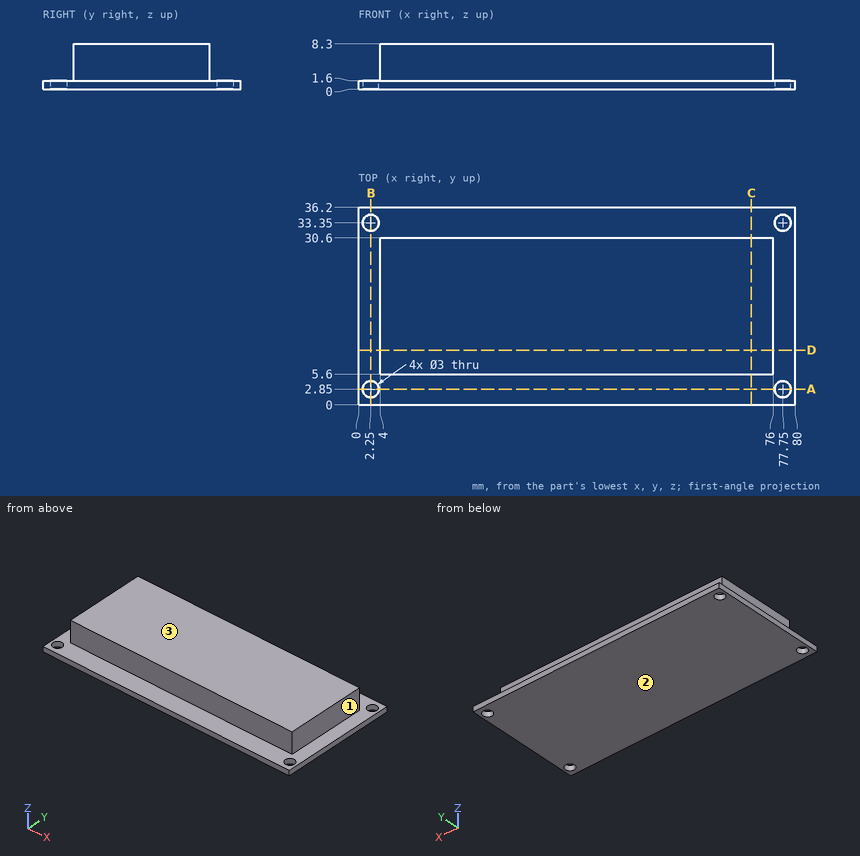
Job drawing, mm, ordinate dimensions from the low corner. One solid piece. Round coordinates to 2 decimals unless told otherwise and drop trailing zeros. Loops run counter-clockwise (first coordinate to the right, second up) from the corner with the lowest first, then second, coordinate; pieces in that order, holes last.
(1) Cut at D-D (y = 10). Give the cut face in (x, z), plus the area to 3 significant figures.
(2) Cut at A-A (y = 2.85). Give the cut face in (x, z).
(3) Drop flat-ended pins along their axis: pin 1 (3.5 mm diameter, centred on x = 2.25, y = 2.85, fed in from +Z); pin 2 (3.5 mm diameter, centred on y = 12.5, z = 3.5, fed in from +X); pin 3 (1 mm diameter, centred on x = 28.5, z = 4.5, fed in from +Y). Give the stop position or say it passes through.
(4) Wall check: line 1 along X through (y, z) = (2.85, 1.3); line 2 along Y through (x, z) = (77.75, 0.65); line 3 along Y through (x, z) = (15, 5.75). Give the ranges that are in metal, low to high.
(5) Cut at B-B (x = 2.25). Give the cut face in (y, z), plus the area to 3 significant figures.
(6) Cut at C-C (x = 72). Give the cut face in (y, z), plus the area to 3 significant figures.
(7) Two-plate mould, pull along Z, no slides. Class the marked faces 1, 2 and 3: +Z half, -Z half, draft (parallel to the pull), parting line (faces both ways), or undercut.
Findings below:
1. outline: (0, 0) - (80, 0) - (80, 1.6) - (76, 1.6) - (76, 8.3) - (4, 8.3) - (4, 1.6) - (0, 1.6) - close
1. area: 610 mm2
2. outline: (0, 0) - (0.75, 0) - (0.75, 1.6) - (0, 1.6) - close; (3.75, 0) - (76.25, 0) - (76.25, 1.6) - (3.75, 1.6) - close; (79.25, 0) - (80, 0) - (80, 1.6) - (79.25, 1.6) - close
3. pin 1: stops at z = 1.6
3. pin 2: stops at x = 76
3. pin 3: stops at y = 30.6
4. line 1: x = 0 to 0.75, 3.75 to 76.25, 79.25 to 80
4. line 2: y = 0 to 1.35, 4.35 to 31.85, 34.85 to 36.2
4. line 3: y = 5.6 to 30.6
5. outline: (0, 0) - (1.35, 0) - (1.35, 1.6) - (0, 1.6) - close; (4.35, 0) - (31.85, 0) - (31.85, 1.6) - (4.35, 1.6) - close; (34.85, 0) - (36.2, 0) - (36.2, 1.6) - (34.85, 1.6) - close
5. area: 48.3 mm2
6. outline: (0, 0) - (36.2, 0) - (36.2, 1.6) - (30.6, 1.6) - (30.6, 8.3) - (5.6, 8.3) - (5.6, 1.6) - (0, 1.6) - close
6. area: 225 mm2
7. face 1: draft
7. face 2: -Z half
7. face 3: +Z half
